The drawing under review shows one solid part. Ordinate dimensions are in mm from its lowest x, y, z. Coordinates: 2 decimals unless noted, no trailing zeros. Write each loop counter-clockwise with the first axis right and the second up, starting at its lowest first coordinate (ties: lowest second). Pieces come first, ordered by that corner, then holes.
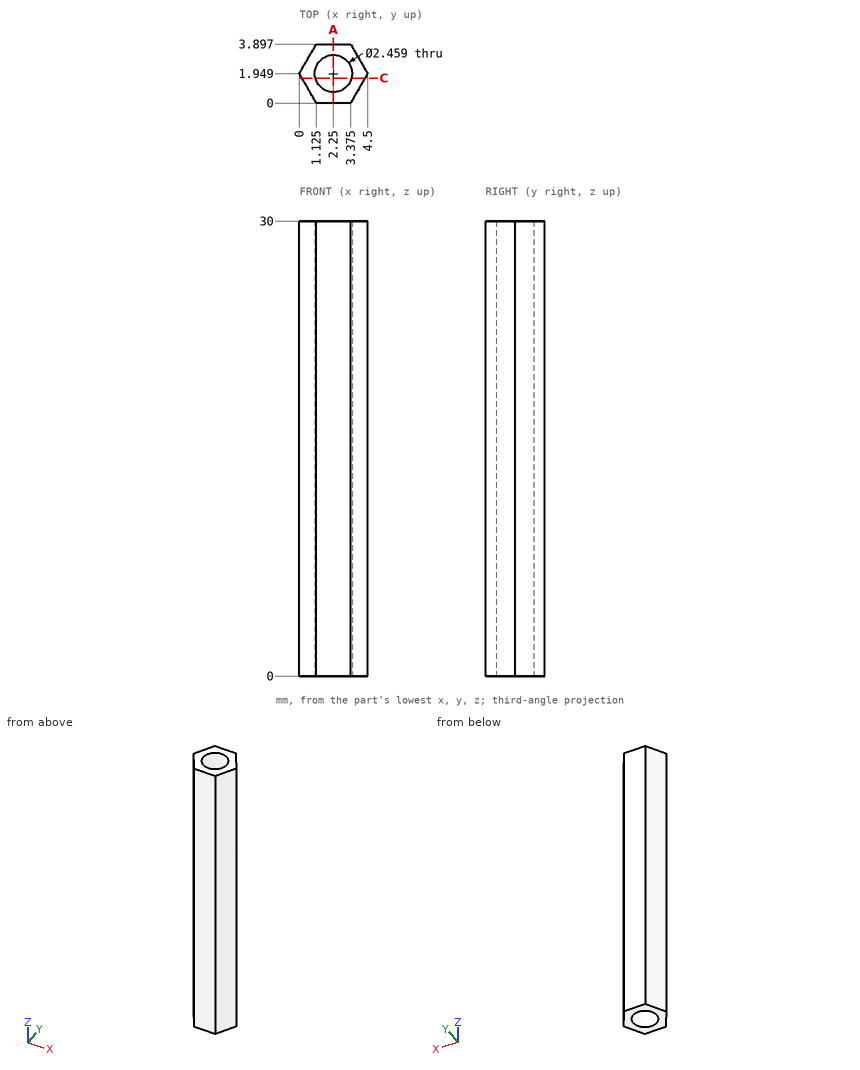
Q1. For probe 1 along Y at (x, z) = (2.2, 14.25); probe 2 along Y at (x, z) = (1.6, 19.5) (1 decimal); probe 3 along X at (y, z) = (1.2, 9.5) (1 decimal), list the stretches that pass through material, from the lowest coordinate up.
Ans:
probe 1: y = 0 to 0.72, 3.18 to 3.9
probe 2: y = 0 to 0.9, 3 to 3.9
probe 3: x = 0.4 to 1.3, 3.2 to 4.1
Q2. Add section C-C (y = 1.65). State the section outline as (x, z) points.
Ans:
outline: (0.17, 0) - (1.06, 0) - (1.06, 30) - (0.17, 30) - close; (3.44, 0) - (4.33, 0) - (4.33, 30) - (3.44, 30) - close
Q3. Add section A-A (x = 2.25). State the section outline as (y, z) points.
Ans:
outline: (0, 0) - (0.72, 0) - (0.72, 30) - (0, 30) - close; (3.18, 0) - (3.9, 0) - (3.9, 30) - (3.18, 30) - close
Q4. Clearance check with flat-ended pins moving along their axes: pin 1 Ø1 at (x, z) = (3.5, 21) entering from -Y; pin 2 Ø1.5 at (x, y) = (2.25, 1.95) entering from +Z; pin 3 Ø1 at (x, z) = (0.5, 18.5) entering from +Y. State where each tip first meets the part, or that it passes through.
Ans:
pin 1: stops at y = 0
pin 2: passes through
pin 3: stops at y = 3.68
